Can you work these out from the drawing? Everything is in mm from the part's minimum corner. Give positions to 0.01 mm unless a question says otherwise; leave off trailing zeros. Write each loop counter-clockwise with the first axis right and the second up, starting at its lowest first coordinate (ties: lowest second). Pieces come first, ordered by that corner, then holes. Notation, with made-up numbers: (73, -13.75) - (116, -13.75) arc R35 cw to (116, 25.25) - close; hole circle Ø9 at (36, -37.75). An arc over 180 degrees is marked (long way). Answer in a Markdown table with one row per item.
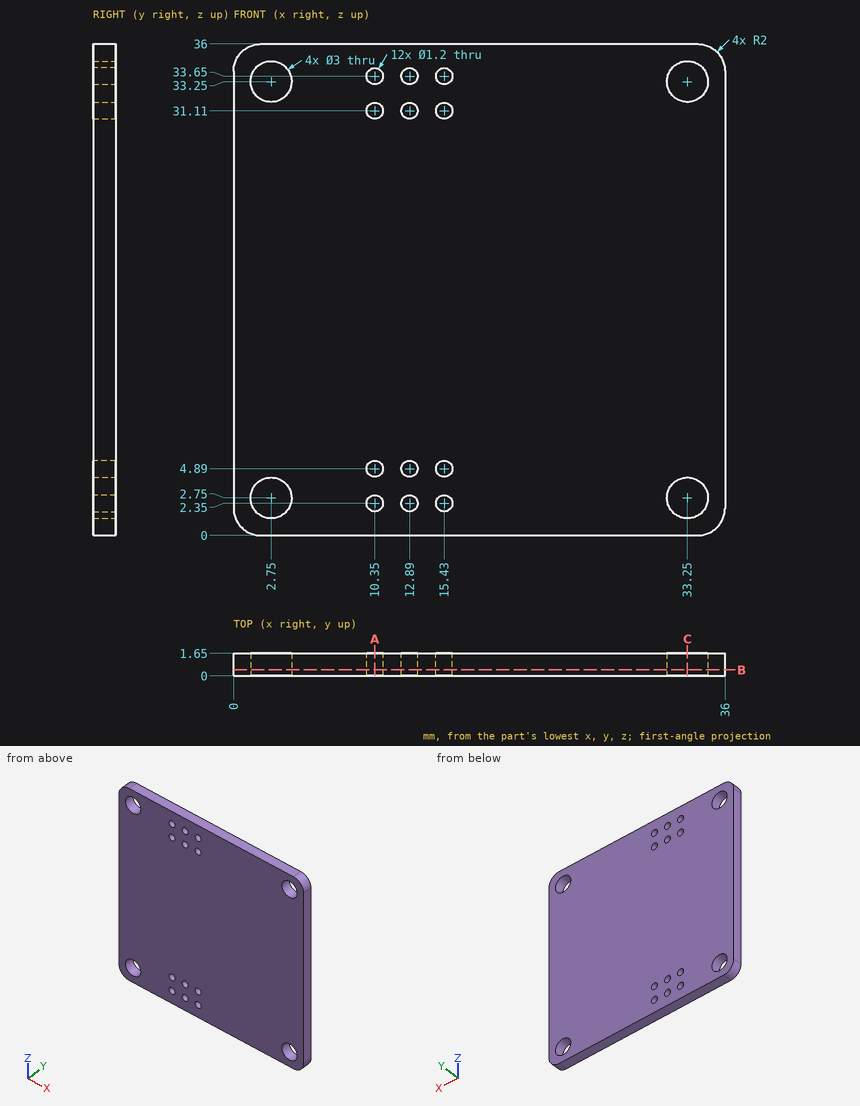
1) Imagine slicing it at C-C (x = 33.25). List the corners of the cut face in (y, z) for me.
Check values:
| item | result |
|---|---|
| outline | (0, 0) - (1.65, 0) - (1.65, 1.25) - (0, 1.25) - close; (0, 4.25) - (1.65, 4.25) - (1.65, 31.75) - (0, 31.75) - close; (0, 34.75) - (1.65, 34.75) - (1.65, 36) - (0, 36) - close |
2) Will this pin go through, and if not, where does the flat tip stop? P1, Ø0.7, axis at x = 12.89, z = 33.65, coming from the -Y side.
Check values:
| item | result |
|---|---|
| P1 | passes through |
3) Imagine slicing it at B-B (y = 0.45). State how many separate pieces and enclosed holes the cut face has, then the cut area to 3 significant figures.
Check values:
| item | result |
|---|---|
| separate pieces | 1 |
| enclosed holes | 16 |
| area | 1,250 mm2 |
4) Imagine slicing it at A-A (x = 10.35). List the corners of the cut face in (y, z) for me, then the cut area to 3 significant figures.
Check values:
| item | result |
|---|---|
| outline | (0, 0) - (1.65, 0) - (1.65, 1.75) - (0, 1.75) - close; (0, 2.95) - (1.65, 2.95) - (1.65, 4.29) - (0, 4.29) - close; (0, 5.49) - (1.65, 5.49) - (1.65, 30.51) - (0, 30.51) - close; (0, 31.71) - (1.65, 31.71) - (1.65, 33.05) - (0, 33.05) - close; (0, 34.25) - (1.65, 34.25) - (1.65, 36) - (0, 36) - close |
| area | 51.5 mm2 |
5) If I drill on line 1 (Z direction, x = 15.5, y = 0.7); line 2 (X direction, y = 1.5, z = 2); line 3 (X direction, y = 0.5, z = 32), over which ranges is the centre line in solid material (lowest first)?
Check values:
| item | result |
|---|---|
| line 1 | z = 0 to 1.75, 2.95 to 4.29, 5.49 to 30.51, 31.71 to 33.05, 34.25 to 36 |
| line 2 | x = 0 to 1.45, 4.05 to 9.86, 10.84 to 12.4, 13.38 to 14.94, 15.92 to 31.95, 34.55 to 36 |
| line 3 | x = 0 to 1.92, 3.58 to 32.42, 34.08 to 36 |
